from build123d import *

# Parameters (mm, degrees)
F0_W          = 80
F0_H          = 80
F0_R          = 23.5
F1_DEPTH      = 40
F1_DEPTH_BACK = 20


with BuildPart() as f1:
    # F0 (on Top) → F1 (new body, two sides)
    with BuildSketch(Plane.XY) as f1_sk:
        Rectangle(F0_W, F0_H)
        Circle(F0_R, mode=Mode.SUBTRACT)
    extrude(amount=F1_DEPTH)
    extrude(f1_sk.sketch, amount=-F1_DEPTH_BACK)


solid = f1.part
Build history of the part. All positions in model axes, mm. Round coordinates to 2 decimals unless told otherwise and drop trailing zeros. Loops run counter-clockwise (first coordinate to the right, second up) from the corner with the lowest first, then second, coordinate; pieces in that order, holes last. Notation, with made-up numbers: (72.5, 32) -> (80.5, 32) arc R14 cw to (80.5, 48) -> close; hole circle Ø10 at (-25.5, -25.5). An arc over 180 degrees is marked (long way). Use CSV: the item, a comma, the result in double quotes. Start each with the question number.
Q1. Mould opens along X. For faces 1 (the face through (-40, -1, 10)), 2 (the face through (22.4, 7.1, 9.6)), 3 (the face through (17, 18, -20)) say: +X half, -X half, draft (parallel to the pull), parting line (faces both ways), or undercut.
Q2. Saw through at C-C on z = -5. Give the cut face in (x, y).
Q3. Drill centre lines: L1, parallel to X at y = -1, z = 8.5; L2, parallel to Y at x = 0, z = -1.5; L3, parallel to Y at x = 18, z = -0.5. Where is each one in solid material? Low to high.
Q4. Saw through at A-A on x = 0. Give the cut face in (y, z), and give its area (3 significant figures).
Solutions:
1,face 1,"-X half"
1,face 2,"undercut"
1,face 3,"draft"
2,outline,"(-40, -40) -> (40, -40) -> (40, 40) -> (-40, 40) -> close; hole circle Ø47 at (0, 0)"
3,L1,"x = -40 to -23.48, 23.48 to 40"
3,L2,"y = -40 to -23.5, 23.5 to 40"
3,L3,"y = -40 to -15.11, 15.11 to 40"
4,outline,"(-40, -20) -> (-23.5, -20) -> (-23.5, 40) -> (-40, 40) -> close; (23.5, -20) -> (40, -20) -> (40, 40) -> (23.5, 40) -> close"
4,area,"1,980 mm^2"
